```python
from build123d import *

# Parameters (mm, degrees)
F0_W           = 40
F0_H           = 30
F1_DEPTH       = 3
F3_D           = 3.2
F4_D           = 5.1
F4_CSINK_D     = 8.96
F4_CSINK_ANGLE = 90
F5_R           = 5


with BuildPart() as f1:
    # F0 (on Front) → F1 (new body)
    with BuildSketch(Plane.XZ):
        Rectangle(F0_W, F0_H)
    extrude(amount=-F1_DEPTH)

    # F3 (through all)
    with Locations(Plane.XZ):
        with Locations((-11, 7.5), (-11, -7.5), (11, 7.5), (11, -7.5)):
            Hole(F3_D / 2)

    # F4 (through all)
    with Locations(Plane.XZ):
        with Locations((-15, 0), (15, 0)):
            CounterSinkHole(F4_D / 2, F4_CSINK_D / 2, counter_sink_angle=F4_CSINK_ANGLE)

    # F5
    f5_edges = [f1.edges().sort_by_distance(p)[0] for p in [
        (20, 1.5, 15),
        (20, 1.5, -15),
        (-20, 1.5, -15),
        (-20, 1.5, 15),
    ]]
    fillet(f5_edges, radius=F5_R)


solid = f1.part
```
Geometry: final body of the model. Coordinates: model frame, mm. Round coordinates to 2 decimals unless told otherwise and drop trailing zeros. Order: outer loops, then holes, each group sorted by start corner. A loop starts at its lowest first (then second) coordinate and runs counter-clockwise, first axis right, second up. Notation, with made-up numbers: (-29.75, 63.5) -> (24.25, 63.5) arc R26 cw to (24.25, 87.5) -> close; hole circle Ø7 at (8, 53). An arc over 180 degrees is marked (long way). Write each question's results on one line, items separated by ' | '.
Q1. Pull-direction query (X, two-part tool) for faces 1 (the face through (12.27, 1.52, 6.53)), 2 (the face through (0, 3, 0)), 3 (the face through (20, 1, 0)); classes: released by +X, released by -X, zero draft, split by the parting line, or undercut.
Response values:
face 1: undercut | face 2: zero draft | face 3: released by +X
Q2. Section query D-D (x = 11.5). Count the separate pieces of the cut face and the enclosed holes in it, and give its area (3 significant figures).
Response values:
separate pieces: 3 | enclosed holes: 0 | area: 68.2 mm²
Q3. Section query A-A (y = 0.8). Output: boundary loops of the cut face in (x, z), and give its area (3 significant figures).
Response values:
outline: (-20, -10) arc R5 ccw to (-15, -15) -> (15, -15) arc R5 ccw to (20, -10) -> (20, 10) arc R5 ccw to (15, 15) -> (-15, 15) arc R5 ccw to (-20, 10) -> close; hole circle Ø7.36 at (-15, 0); hole circle Ø3.2 at (-11, -7.5); hole circle Ø3.2 at (-11, 7.5); hole circle Ø3.2 at (11, -7.5); hole circle Ø3.2 at (11, 7.5); hole circle Ø7.36 at (15, 0) | area: 1,060 mm²
Q4. Section query C-C (z = 7.5). Output: boundary loops of the cut face in (x, y).
Response values:
outline: (-20, 0) -> (-12.6, 0) -> (-12.6, 3) -> (-20, 3) -> close; (-9.4, 0) -> (9.4, 0) -> (9.4, 3) -> (-9.4, 3) -> close; (12.6, 0) -> (20, 0) -> (20, 3) -> (12.6, 3) -> close
Q5. Section query B-B (z = 0). Output: boundary loops of the cut face in (x, y), and give its area (4 significant figures).
Response values:
outline: (-20, 0) -> (-19.48, 0) -> (-17.55, 1.93) -> (-17.55, 3) -> (-20, 3) -> close; (-12.45, 1.93) -> (-10.52, 0) -> (10.52, 0) -> (12.45, 1.93) -> (12.45, 3) -> (-12.45, 3) -> close; (17.55, 1.93) -> (19.48, 0) -> (20, 0) -> (20, 3) -> (17.55, 3) -> close | area: 81.95 mm²
Q6. Ray query, line 1 along Z through (x, y) = (-11, 1.9); line 2 along X through (y, z) = (2.45, 0); line 3 along X through (y, z) = (2.7, 1). Return the intervals inside material, ascending.
Response values:
line 1: -15 to -9.1, -5.9 to 5.9, 9.1 to 15 | line 2: -20 to -17.55, -12.45 to 12.45, 17.55 to 20 | line 3: -20 to -17.35, -12.65 to 12.65, 17.35 to 20
